```python
from build123d import *

# Parameters (mm, degrees)
SKETCH_1_R          = 2.5
EXTRUDE_1_DEPTH     = 12
SKETCH_2_R          = 3.635
EXTRUDE_2_DEPTH     = 2
SKETCH_3_W          = 10.772084644
SKETCH_3_H          = 1
CUT_EXTRUDE_1_DEPTH = 1
SKETCH_4_W          = 1
SKETCH_4_H          = 4.75
CUT_EXTRUDE_2_DEPTH = 1


with BuildPart() as part:
    # 草图1 → 拉伸1 (new body)
    with BuildSketch(Plane(origin=(0, 0, 0), x_dir=(1, 0, 0), z_dir=(0, 1, 0))):
        with Locations(Location((0, 0, 0), (0, 0, 270))):
            Circle(SKETCH_1_R)
    extrude(amount=EXTRUDE_1_DEPTH)

    # 草图2 → 拉伸2 (add)
    with BuildSketch(Plane(origin=(0, 12, 0), x_dir=(-1, 0, 0), z_dir=(0, 1, 0))):
        with Locations(Location((0, 0, 0), (0, 0, 90))):
            Circle(SKETCH_2_R)
    extrude(amount=EXTRUDE_2_DEPTH)

    # 草图3 → 切除-拉伸1 (cut)
    with BuildSketch(Plane(origin=(0, 14, 0), x_dir=(-1, 0, 0), z_dir=(0, 1, 0))):
        Rectangle(SKETCH_3_W, SKETCH_3_H)
    extrude(amount=-CUT_EXTRUDE_1_DEPTH, mode=Mode.SUBTRACT)

    # 草图4 → 切除-拉伸2 (cut)
    with BuildSketch(Plane(origin=(0, 14, 0), x_dir=(-1, 0, 0), z_dir=(0, 1, 0))):
        Rectangle(SKETCH_4_W, SKETCH_4_H)
    extrude(amount=-CUT_EXTRUDE_2_DEPTH, mode=Mode.SUBTRACT)

    # 草图5 → 切除-旋转16 (revolve, cut)
    with BuildSketch(Plane(origin=(0, 0, 0), x_dir=(0, 0, -1), z_dir=(1, 0, 0)), mode=Mode.PRIVATE) as cut_revolve_16_sk:
        with BuildLine():
            Line((0, 14.65344885), (-4.227714807, 14.65344885))
            Line((-4.227714807, 14.65344885), (-4.227714807, 12.257514241))
            ThreePointArc((-4.227714807, 12.257514241), (-2.28636333, 13.54730049), (0, 14))
            Line((0, 14), (0, 14.65344885))
        make_face()
    revolve(cut_revolve_16_sk.sketch.rotate(Axis((0, -2.105917543, 0), (0, 1, 0)), 180), axis=Axis((0, -2.105917543, 0), (0, 1, 0)), mode=Mode.SUBTRACT)


solid = part.part
```
Design review of the part built by this model. Coordinates are the model's own, in mm. A direction names the side the tool comes from. Coordinates: 2 decimals unless noted, no trailing zeros. Write each loop counter-clockwise with the first axis right and the second up, starting at its lowest first coordinate (ties: lowest second). Pieces come first, ordered by that corner, then holes. Notation, with made-up numbers: M 35,68.5 L 60,68.5 A15 cw 60,80.5 Z; hole C -37,35.25 d8. An arc over 180 degrees is marked long. Answer as a JSON object with one key per item and string values.
Item 1: Insertion check: pin 1 Ø1.1 at (x, y) = (-2, 13.5) entering from +Z; pin 2 Ø0.8 at (y, z) = (13.5, 2) entering from +X; pin 3 Ø3 at (x, y) = (2.5, 6.5) entering from +Z. Each pin has a flat end and moves straight along its axis. Give the tip position at first contact, or say it passes through.
Outcome:
{"pin 1": "z = 2.81", "pin 2": "x = 2.5", "pin 3": "z = 2.29"}
Item 2: Add section C-C, the plane y = 6.25. Give the boundary of the cut face in (x, z), and give its area (3 significant figures).
Outcome:
{"outline": "C 0,0 d5", "area": "19.6 mm²"}
Item 3: Add section A-A, the plane z = 0. Give the boundary of the cut face in (x, y) (3 decimals).
Outcome:
{"outline": "M -3.635,12 L -2.5,12 L -2.5,0 L 2.5,0 L 2.5,12 L 3.635,12 L 3.635,12.774 A6 ccw 3.317,13 L -3.317,13 A6 ccw -3.635,12.774 Z"}
Item 4: Add section D-D, the plane z = -1.25. Give the boundary of the cut face in (x, y), and give its area (3 significant figures).
Outcome:
{"outline": "M -3.41,12 L -2.17,12 L -2.17,0 L 2.17,0 L 2.17,12 L 3.41,12 L 3.41,12.77 A5.87 ccw 0.5,13.85 L 0.5,13 L -0.5,13 L -0.5,13.85 A5.87 ccw -3.41,12.77 Z", "area": "61.5 mm²"}
Item 5: Wall thickness on probe 1 along X at (y, z) = (9.5, 0); probe 2 along Y at (x, z) = (2, -3); probe 3 along X at (y, z) = (7, 1.5): over which ranges is each line inside the solid? List them lowest first.
Outcome:
{"probe 1": "-2.5 to 2.5", "probe 2": "12 to 12.8", "probe 3": "-2 to 2"}
Item 6: Add section B-B, the plane x = 0. Give the boundary of the cut face in (y, z) (3 decimals), and give its area (3 significant figures).
Outcome:
{"outline": "M 0,-2.5 L 12,-2.5 L 12,-3.635 L 12.774,-3.635 A6 ccw 13.51,-2.375 L 13,-2.375 L 13,2.375 L 13.51,2.375 A6 ccw 12.774,3.635 L 12,3.635 L 12,2.5 L 0,2.5 Z", "area": "67.7 mm²"}
Item 7: Draft analysis for pull direction Z (two halves, no side actions). For faces 5 (the flat face through (2.5, 12, -0.9)), 6 (the flat face through (0.5, 13.4, -1.5)), 7 (the cylindrical face through (-2.212, 12.381, -2.885)), state which applies: pulls with the +Z half, pulls with the -Z half, needs draft (parallel to the pull), parting line crosses it, or undercut.
Outcome:
{"face 5": "needs draft", "face 6": "undercut", "face 7": "parting line crosses it"}
Item 8: Machinability: for faces 1 (the cylindrical face through (-2.44, 5.92, -0.54)), 2 (the flat face through (-0.5, 13.4, -1.5)), 3 (the flat face through (0, 0, 0)), 4 (the flat face through (-1.6, 13.4, -0.5)), which of the approach directions +Z, -Z, +X, -X, +Y, -Y give a long, thin tool a straight path to every point of the face, cutting with its end or side? Answer none if there is none.
Outcome:
{"face 1": "-Y", "face 2": "+Y", "face 3": "+Z, -Z, +X, -X, -Y", "face 4": "+X, -X, +Y"}
